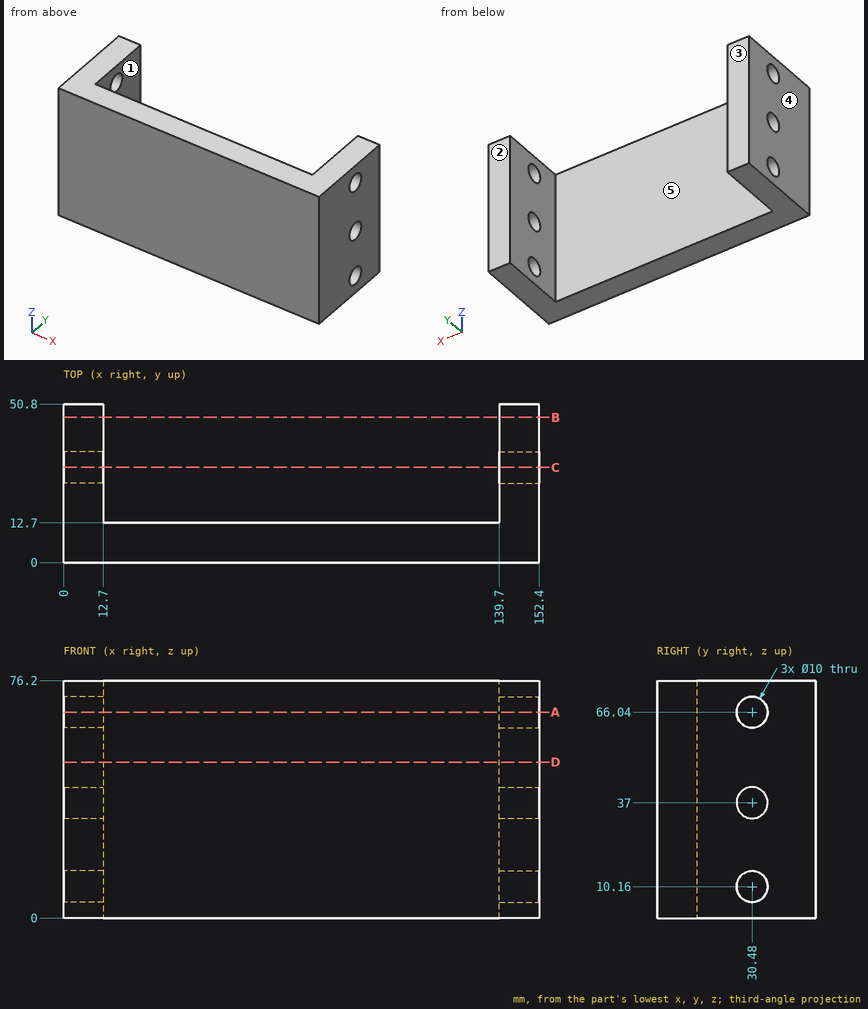
Geometry: see drawing. Coordinates: mm, zero at the bounding-box minimum. A direction names the side the tool comes from. Give positions to 0.01 mm unless a question says otherwise; leave off trailing zeros. Write each loop counter-clockwise with the first axis right and the second up, starting at its lowest first coordinate (ties: lowest second). Pieces come first, ordered by that corner, then holes. Notation, with made-up numbers: M 47,33.5 L 97,33.5 A26 cw 97,69.5 Z; hole C -9.5,67.25 d6. An arc over 180 degrees is marked long. Return JSON: item names as keys, results as strings. Group by question number.
1) Cut plane A-A, the plane z = 66.04. Output: boundary loops of the cut face in (x, y).
2) Cut plane C-C, the plane y = 30.48. Give the number of separate pieces and of enclosed holes in the cut face, then the cut area to 3 significant figures.
3) First-contact query: pin 1 Ø3 at (x, z) = (106.5, 61) entering from +Y; pin 2 Ø6 at (y, z) = (30.48, 66.04) entering from +X. Flat tips, straight axial feed; report the tip coordinate or a pass-through.
4) Cut plane B-B, the plane y = 46.5. Output: boundary loops of the cut face in (x, z).
5) Cut plane D-D, the plane z = 50. Output: boundary loops of the cut face in (x, y), then the cut area to 3 significant figures.
6) Ray query, L1, parallel to Z at x = 148, y = 30; L2, parallel to Z at x = 149.25, y = 30.48; L3, parallel to X at y = 16, z = 56. Return the intervals inside material, ascending.
7) Draft query along X for the marked faces 3, 4 and 5. Return one class per face: released by +X, released by -X, zero draft, split by the parting line, or undercut.
8) Set-up query: the marked faces 1 and 2. Return all of +Z, -Z, +X, -X, +Y, -Y with unobstructed straight access to the full face (end or side cutting, diameter ignored); none if empty.
Data:
{
 "1": {"outline": "M 0,0 L 152.4,0 L 152.4,25.48 L 139.7,25.48 L 139.7,12.7 L 12.7,12.7 L 12.7,25.48 L 0,25.48 Z; M 0,35.48 L 12.7,35.48 L 12.7,50.8 L 0,50.8 Z; M 139.7,35.48 L 152.4,35.48 L 152.4,50.8 L 139.7,50.8 Z"},
 "2": {"separate pieces": "8", "enclosed holes": "0", "area": "1,170 mm²"},
 "3": {"pin 1": "stops at y = 12.7", "pin 2": "passes through"},
 "4": {"outline": "M 0,0 L 12.7,0 L 12.7,76.2 L 0,76.2 Z; M 139.7,0 L 152.4,0 L 152.4,76.2 L 139.7,76.2 Z"},
 "5": {"outline": "M 0,0 L 152.4,0 L 152.4,50.8 L 139.7,50.8 L 139.7,12.7 L 12.7,12.7 L 12.7,50.8 L 0,50.8 Z", "area": "2,900 mm²"},
 "6": {"L1": "z = 0 to 5.18, 15.14 to 32.02, 41.98 to 61.06, 71.02 to 76.2", "L2": "z = 0 to 5.16, 15.16 to 32, 42 to 61.04, 71.04 to 76.2", "L3": "x = 0 to 12.7, 139.7 to 152.4"},
 "7": {"face 3": "zero draft", "face 4": "released by -X", "face 5": "undercut"},
 "8": {"face 1": "+Z, -Z, +Y", "face 2": "+Z, -Z, +X, -X, +Y"}
}
